```python
from build123d import *

# Parameters (mm, degrees)
EXTRUDE_1_DEPTH = 4


with BuildPart() as part:
    # Эскиз1 → Бобышка-Вытянуть1 (new body)
    with BuildSketch(Plane(origin=(0, 0, 0), x_dir=(1, 0, 0), z_dir=(0, 1, 0))):
        with BuildLine():
            Line((10, -17.5), (2, -17.5))
            Line((2, -17.5), (2, -20.5))
            Line((2, -20.5), (4, -20.5))
            Line((4, -20.5), (4, -22.5))
            Line((4, -22.5), (-4, -22.5))
            Line((-4, -22.5), (-4, -20.5))
            Line((-4, -20.5), (-2, -20.5))
            Line((-2, -20.5), (-2, -17.5))
            Line((-2, -17.5), (-10, -17.5))
            Line((-10, -17.5), (-10, -7.5))
            ThreePointArc((-10, -7.5), (-7.461085915, 4.585557713), (-1.607525862, 15.459500175))
            ThreePointArc((-1.607525862, 15.459500175), (0, 16.269600766), (1.607525862, 15.459500175))
            ThreePointArc((1.607525862, 15.459500175), (7.461085915, 4.585557713), (10, -7.5))
            Line((10, -7.5), (10, -17.5))
        make_face()
    extrude(amount=EXTRUDE_1_DEPTH)


solid = part.part
```
Check sheet for the modelled part. Datum: model origin and axes. Units: mm. A direction names the side the tool comes from. Give positions to 0.01 mm unless a question says otherwise; leave off trailing zeros. Write each loop counter-clockwise with the first axis right and the second up, starting at its lowest first coordinate (ties: lowest second). Pieces come first, ordered by that corner, then holes. Notation, with made-up numbers: (11.25, 65.25) - (51.25, 65.25) arc R25 cw to (51.25, 99.25) - close; hole circle Ø5 at (58.25, -24.5). An arc over 180 degrees is marked (long way). Answer as a JSON object with one key per item and string values. Group by question number.
1) Sectioned sample at C-C (z = 1). Record the cut outline in (x, y), then the cut area to 3 significant figures.
2) Depth check by flat-ended pin: P1, Ø0.6, axis at x = 2.5, y = 2.5, coming from the -Z side; P2, Ø1, axis at y = 1.5, z = 21, coming from the -X side; P3, Ø1, axis at y = 3, z = 21, coming from the +X side. Enter the tip coordinate at first touch or a pass-through.
3) Thickness scan on probe 1 along Z at (x, y) = (-3.75, 0.8); probe 2 along X at (y, z) = (0.55, 20); probe 3 along X at (y, z) = (2.4, -1.5). Record the ranges inside material, lowest first. Write a range as from..to.
4) Sectioned sample at A-A (x = 2.75). Record the cut outline in (y, z), then the cut area to 3 significant figures.
5) Sectioned sample at D-D (x = -7). Record the cut outline in (y, z).
6) Sectioned sample at B-B (y = 3.55). Record the cut outline in (x, z).
7) Release check for a two-part mould opening along Z. For faces 1 (the face through (0, 2, 22.5)), 2 (the face through (10, 2, 12)), 3 (the face through (2, 2, 19)) record: pulls with the +Z half, pulls with the -Z half, needs draft (parallel to the pull), parting line crosses it, or undercut.
8) Access from +Z, -Z, +X, -X, +Y, -Y to the whole of each face (thin tool, end or side, straight path). Record for faces 4 (the face through (-4, 2, 22)), 5 (the face through (4, 2, 21)), 6 (the face through (-6, 2, 17.5)).
Geometry results:
{
 "1": {"outline": "(-9.09, 0) - (9.09, 0) - (9.09, 4) - (-9.09, 4) - close", "area": "72.7 mm^2"},
 "2": {"P1": "stops at z = -14.64", "P2": "stops at x = -4", "P3": "stops at x = 4"},
 "3": {"probe 1": "z = -12.28..17.5, 20.5..22.5", "probe 2": "x = -2..2", "probe 3": "x = -8.46..8.46"},
 "4": {"outline": "(0, -13.84) - (4, -13.84) - (4, 17.5) - (0, 17.5) - close; (0, 20.5) - (4, 20.5) - (4, 22.5) - (0, 22.5) - close", "area": "133 mm^2"},
 "5": {"outline": "(0, -5.79) - (4, -5.79) - (4, 17.5) - (0, 17.5) - close"},
 "6": {"outline": "(-10, 7.5) arc R43.21 ccw to (-1.61, -15.46) arc R2 ccw to (1.61, -15.46) arc R43.21 ccw to (10, 7.5) - (10, 17.5) - (2, 17.5) - (2, 20.5) - (4, 20.5) - (4, 22.5) - (-4, 22.5) - (-4, 20.5) - (-2, 20.5) - (-2, 17.5) - (-10, 17.5) - close"},
 "7": {"face 1": "pulls with the +Z half", "face 2": "needs draft", "face 3": "undercut"},
 "8": {"face 4": "+Z, -X, +Y, -Y", "face 5": "+Z, +X, +Y, -Y", "face 6": "-X, +Y, -Y"}
}
